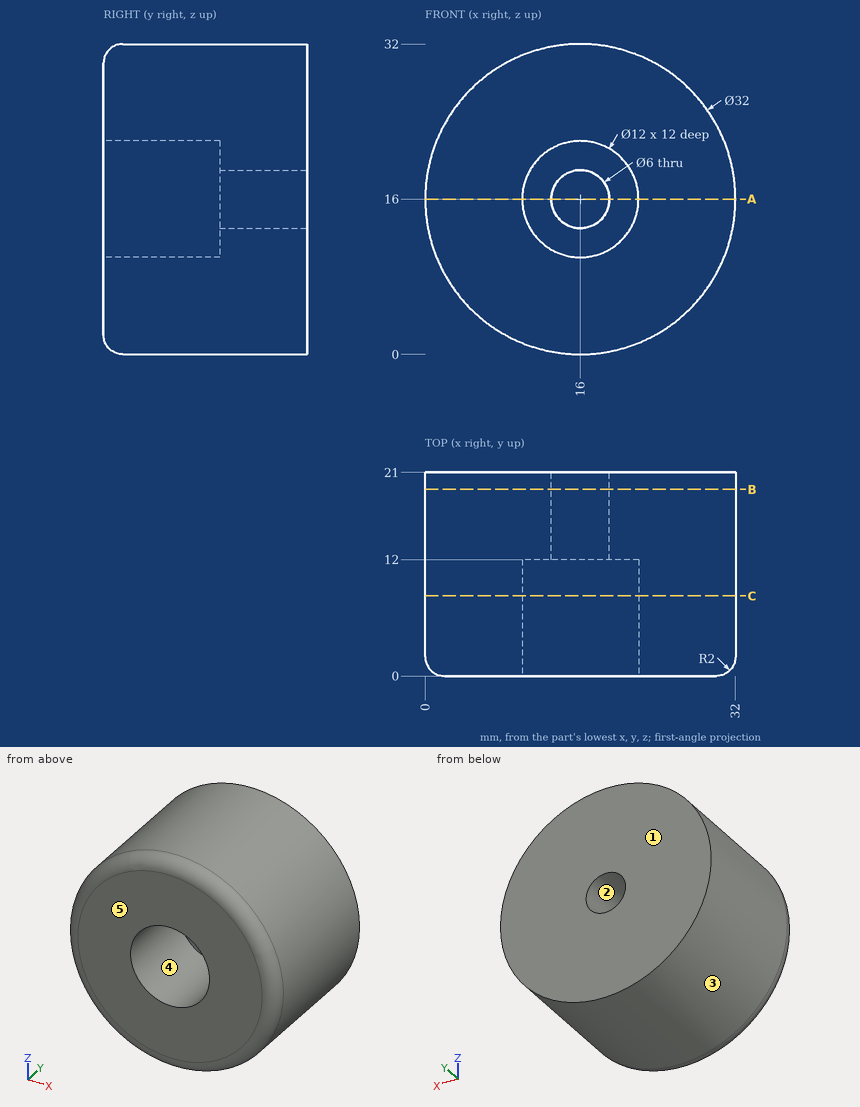
Source: three-view drawing plus pictorial views. Frame: mm from the lowest corner of the part. A direction names the side the tool comes from. Give positions to 0.01 mm unless a question says otherwise; leave off trailing zeros. Order: outer loops, then holes, each group sorted by start corner. A loop starts at its lowest first (then second) coordinate and runs counter-clockwise, first axis right, second up.
1. Section C-C on y = 8.25. Return the cut outline in (x, z), and give its area (3 significant figures).
Derived:
outline: circle Ø32 at (16, 16); hole circle Ø12 at (16, 16)
area: 691 mm2
2. Pin query (flat end, axial travel): pin 1 (1.5 mm diameter, centred on x = 6.5, y = 18.5, fed in from +Z); pin 2 (2 mm diameter, centred on y = 2.5, z = 14, fed in from +X); pin 3 (5 mm diameter, centred on x = 5, y = 18.5, fed in from +Z). Return the tip coordinate at first contact, or that it passes through.
Derived:
pin 1: stops at z = 29.4
pin 2: stops at x = 31.97
pin 3: stops at z = 29.56
3. Mould query, pull axis X, two halves, no side actions, for the marked faces 1, 2 and 3. Classes: released by +X, released by -X, zero draft, split by the parting line, or undercut.
Derived:
face 1: zero draft
face 2: undercut
face 3: split by the parting line
4. Material intervals for L1, parallel to Z at x = 16, y = 19; L2, parallel to Z at x = 16, y = 2.75; L3, parallel to Y at x = 16.5, z = 19.5, sorted ascending.
Derived:
L1: z = 0 to 13, 19 to 32
L2: z = 0 to 10, 22 to 32
L3: y = 12 to 21
5. Reachability of the marked faces 4 and 5 from +Z, -Z, +X, -X, +Y, -Y: full face, straight path, thin tool, end or side. Return the list, or none.
Derived:
face 4: -Y
face 5: +Z, -Z, +X, -X, -Y
6. Section A-A on z = 16. Return the cut outline in (x, y).
Derived:
outline: (0, 2) arc R2 ccw to (2, 0) - (10, 0) - (10, 12) - (13, 12) - (13, 21) - (0, 21) - close; (19, 12) - (22, 12) - (22, 0) - (30, 0) arc R2 ccw to (32, 2) - (32, 21) - (19, 21) - close
7. Section B-B on y = 19.25. Return the cut outline in (x, z).
Derived:
outline: circle Ø32 at (16, 16); hole circle Ø6 at (16, 16)
